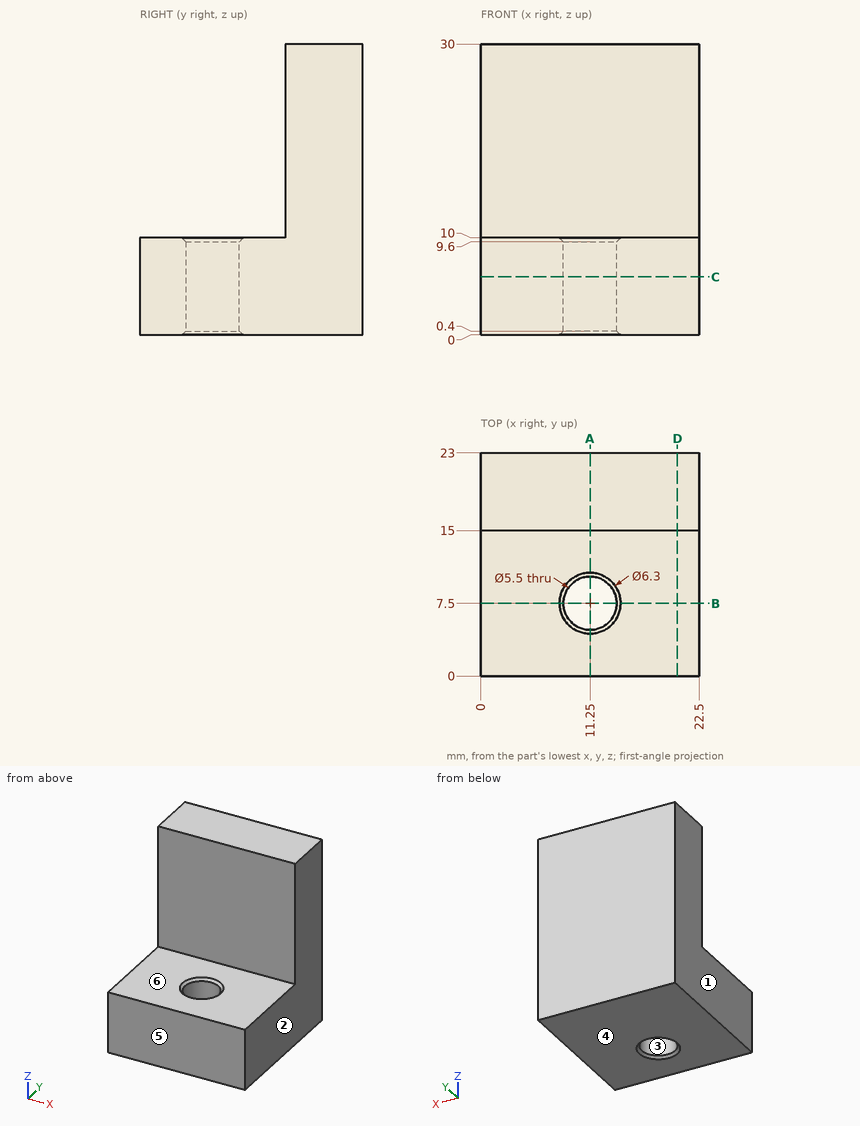
Geometry: see drawing. Coordinates: mm, zero at the bounding-box minimum. A direction names the side the tool comes from. Coordinates: 2 decimals unless noted, no trailing zeros. Write each loop counter-clockwise with the first axis right and the second up, starting at its lowest first coordinate (ties: lowest second). Pieces come first, ordered by that corner, then holes. Notation, with made-up numbers: M -25.5,68 L -9.5,68 A19 ccw -9.5,103 Z; hole C -1.5,37 d4. An arc over 180 degrees is marked long. Use CSV: the item, a comma, the result in double quotes. Start each with the question number.
1. Reachability of the marked faces 5 and 6 from +Z, -Z, +X, -X, +Y, -Y: full face, straight path, thin tool, end or side. Return the list, or none.
2. Cut plane D-D on x = 20.25. Return the cut outline in (y, z), plus the area to 3 significant figures.
3. Cut plane C-C on z = 6. Return the cut outline in (x, y).
4. Cut plane B-B on y = 7.5. Return the cut outline in (x, z), plus the area to 3 significant figures.
5. Mould query, pull axis X, two halves, no side actions, for the marked faces 1, 2, 3 and 4. Classes: pulls with the +X half, pulls with the -X half, needs draft (parallel to the pull), parting line crosses it, or undercut.
6. First-contact query: P1, Ø1, axis at x = 9.5, y = 16, coming from the -Z side; P2, Ø8, axis at x = 19, y = 7.5, coming from the +Z side; P3, Ø6, axis at x = 3.5, z = 16, coming from the -Y side; P4, Ø5, axis at x = 11.25, y = 7.5, coming from the -Z side. Flat tips, straight axial feed; report the tip coordinate or a pass-through.
7. Ray query, probe 1 along Y at (x, z) = (11.25, 2.5); probe 2 along X at (y, z) = (7.5, 5.75); probe 3 along Z at (x, y) = (4.5, 6). Return the intervals inside material, ascending.
8. Cut plane A-A on x = 11.25. Return the cut outline in (y, z).
Entries:
1,face 5,"+Z, -Z, +X, -X, -Y"
1,face 6,"+Z, +X, -X, -Y"
2,outline,"M 0,0 L 23,0 L 23,30 L 15,30 L 15,10 L 0,10 Z"
2,area,"390 mm²"
3,outline,"M 0,0 L 22.5,0 L 22.5,23 L 0,23 Z; hole C 11.25,7.5 d5.5"
4,outline,"M 0,0 L 8.1,0 L 8.5,0.4 L 8.5,9.6 L 8.1,10 L 0,10 Z; M 14,0.4 L 14.4,0 L 22.5,0 L 22.5,10 L 14.4,10 L 14,9.6 Z"
4,area,"170 mm²"
5,face 1,"pulls with the -X half"
5,face 2,"pulls with the +X half"
5,face 3,"undercut"
5,face 4,"needs draft"
6,P1,"z = 0"
6,P2,"z = 10"
6,P3,"y = 15"
6,P4,"through"
7,probe 1,"0 to 4.75, 10.25 to 23"
7,probe 2,"0 to 8.5, 14 to 22.5"
7,probe 3,"0 to 10"
8,outline,"M 0,0 L 4.35,0 L 4.75,0.4 L 4.75,9.6 L 4.35,10 L 0,10 Z; M 10.25,0.4 L 10.65,0 L 23,0 L 23,30 L 15,30 L 15,10 L 10.65,10 L 10.25,9.6 Z"
